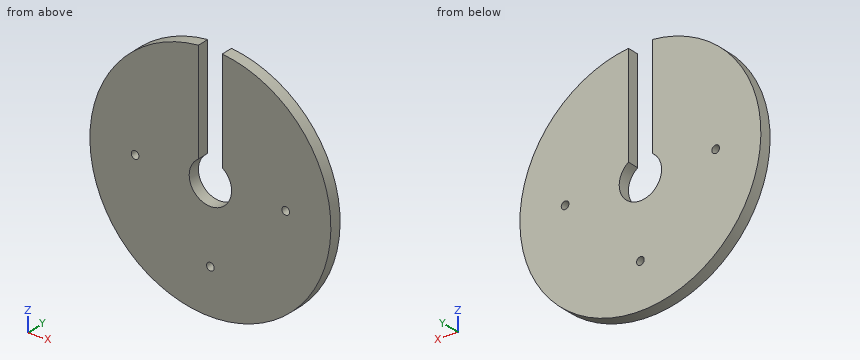
from build123d import *

# Parameters (mm, degrees)
SKETCH1_R           = 101.6
BOSS_EXTRUDE1_DEPTH = 10
SKETCH2_R           = 3.25
CUT_EXTRUDE1_DEPTH  = 145.031663186


with BuildPart() as part:
    # Sketch1 → Boss-Extrude1 (new body)
    with BuildSketch(Plane(origin=(0, 0, 0), x_dir=(1, 0, 0), z_dir=(0, 1, 0))):
        with Locations(Location((0, 0, 0), (0, 0, 270))):
            Circle(SKETCH1_R)
    extrude(amount=BOSS_EXTRUDE1_DEPTH)

    # Sketch2 → Cut-Extrude1 (cut, through all)
    with BuildSketch(Plane(origin=(0, 10, 0), x_dir=(1, 0, 0), z_dir=(0, 1, 0))):
        with Locations(Location((63.5, 0.070795045, 0), (0, 0, 270))):
            Circle(SKETCH2_R)
        with Locations(Location((-63.5, 0.070795045, 0), (0, 0, 270))):
            Circle(SKETCH2_R)
        with Locations(Location((0, 63.570795045, 0), (0, 0, 270))):
            Circle(SKETCH2_R)
        with BuildLine():
            Line((10, -14.746676337), (10, -101.106676337))
            ThreePointArc((10, -101.106676337), (0, -101.6), (-10, -101.106676337))
            Line((-10, -101.106676337), (-10, -14.746676337))
            ThreePointArc((-10, -14.746676337), (0, 17.946965165), (10, -14.746676337))
        make_face()
    extrude(amount=-CUT_EXTRUDE1_DEPTH, mode=Mode.SUBTRACT)


solid = part.part
Input: part model. Units: mm. Frame: model coordinates. Coordinates: 2 decimals unless noted, no trailing zeros. Loops run counter-clockwise (first coordinate to the right, second up) from the corner with the lowest first, then second, coordinate; pieces in that order, holes last. Notation, with made-up numbers: (6.5, -13.75) -> (10.5, -13.75) arc R25 ccw to (10.5, 11.25) -> close; hole circle Ø9 at (62, 2). An arc over 180 degrees is marked (long way). Write item = value, one per line. Start each with the question number.
Item 1: Cut plane C-C, the plane z = 25.5. Return loops of the section in (x, y), plus the area to 3 significant figures.
Item 2: Material intervals for line 1 (Z direction, x = 64.5, y = 3.25); line 2 (Z direction, x = 1.5, y = 2.5); line 3 (X direction, y = 4, z = 26), sorted ascending.
Item 3: First-contact query: P1, Ø4, axis at x = 63.5, z = -0.07, coming from the +Y side; P2, Ø1, axis at y = 8.5, z = 33, coming from the -X side; P3, Ø6, axis at x = -22, y = 6, coming from the -Z side; P4, Ø4, axis at x = 26, y = 5.5, coming from the +Z side. Flat tips, straight axial feed; report the tip coordinate or a pass-through.
Item 4: Cut plane D-D, the plane z = 0. Return loops of the section in (x, y), plus the area to 3 significant figures.
Item 5: Cut plane A-A, the plane x = 0. Return loops of the section in (y, z), plus the area to 3 significant figures.
Item 6: Cut plane B-B, the plane y = 5.5. Return loops of the section in (x, z).
Ans:
q1.outline = (-98.35, 0) -> (-10, 0) -> (-10, 10) -> (-98.35, 10) -> close; (10, 0) -> (98.35, 0) -> (98.35, 10) -> (10, 10) -> close
q1.area = 1,770 mm²
q2.line_1 = -78.5 to -3.16, 3.02 to 78.5
q2.line_2 = -101.59 to -66.45, -60.69 to -17.88
q2.line_3 = -98.22 to -10, 10 to 98.22
q3.P1 = through
q3.P2 = -96.26
q3.P3 = -99.81
q3.P4 = 98.72
q4.outline = (-101.6, 0) -> (-66.75, 0) -> (-66.75, 10) -> (-101.6, 10) -> close; (-60.25, 0) -> (-17.88, 0) -> (-17.88, 10) -> (-60.25, 10) -> close; (17.88, 0) -> (60.25, 0) -> (60.25, 10) -> (17.88, 10) -> close; (66.75, 0) -> (101.6, 0) -> (101.6, 10) -> (66.75, 10) -> close
q4.area = 1,540 mm²
q5.outline = (0, -101.6) -> (10, -101.6) -> (10, -66.82) -> (0, -66.82) -> close; (0, -60.32) -> (10, -60.32) -> (10, -17.95) -> (0, -17.95) -> close
q5.area = 772 mm²
q6.outline = (-10, 14.75) -> (-10, 101.11) arc R101.6 ccw (long way) to (10, 101.11) -> (10, 14.75) arc R17.88 cw (long way) to start; hole circle Ø6.5 at (-63.5, -0.07); hole circle Ø6.5 at (0, -63.57); hole circle Ø6.5 at (63.5, -0.07)
